Design review of the part built by this model. Coordinates are the model's own, in mm. Coordinates: 2 decimals unless noted, no trailing zeros. Order: outer loops, then holes, each group sorted by start corner. A loop starts at its lowest first (then second) coordinate and runs counter-clockwise, first axis right, second up. Notation, with made-up numbers: (24.25, 81) -> (82.25, 81) arc R19 ccw to (82.25, 114) -> close; hole circle Ø7 at (-13.5, 16.25). An arc over 180 degrees is marked (long way). Write item = value, one per line.
```python
from build123d import *

# Parameters (mm, degrees)
BOSS_EXTRUDE1_DEPTH = 6.35
SKETCH2_R           = 6.35
CUT_EXTRUDE1_DEPTH  = 6.35
CUT_EXTRUDE4_DEPTH  = 6.35


with BuildPart() as part:
    # Sketch1 → Boss-Extrude1 (new body)
    with BuildSketch(Plane.XY):
        Polygon((20.505148302, 25.897062134), (-23.613528139, 31.314154449), (25.914173021, 434.684910476), (95.764173021, 434.684910476), (95.764173021, 95.747062134), (29.081649881, 95.747062134), align=None)
    extrude(amount=BOSS_EXTRUDE1_DEPTH)

    # Sketch2 → Cut-Extrude1 (cut)
    with BuildSketch(Plane.XY.offset(6.35)):
        with Locations((72.594859494, 436.135448726)):
            Circle(SKETCH2_R)
    extrude(amount=-CUT_EXTRUDE1_DEPTH, mode=Mode.SUBTRACT)

    # Sketch4 → Cut-Extrude4 (cut)
    with BuildSketch(Plane.XY.offset(6.35)):
        with BuildLine():
            Line((74.295018445, 431.943320697), (82.016159891, 440.361424689))
            Line((82.016159891, 440.361424689), (105.989857785, 438.164600241))
            Line((105.989857785, 438.164600241), (95.764173021, 334.935994434))
            ThreePointArc((95.764173021, 334.935994434), (92.231289046, 356.088107858), (82.016159891, 374.943990437))
            ThreePointArc((82.016159891, 374.943990437), (70.461962448, 402.401475249), (74.295018445, 431.943320697))
        make_face()
    extrude(amount=-CUT_EXTRUDE4_DEPTH, mode=Mode.SUBTRACT)


solid = part.part
```
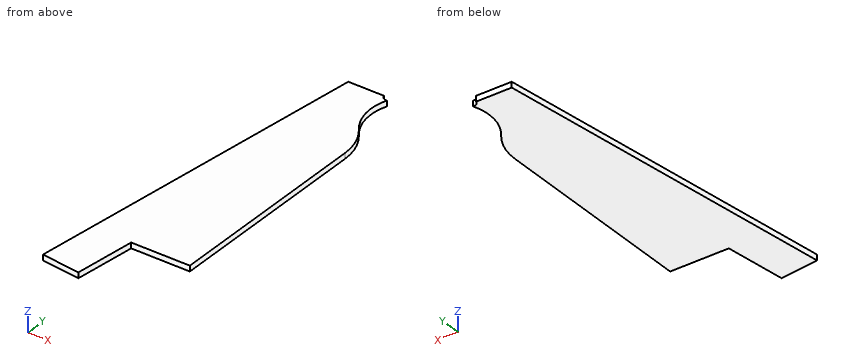
(1) Insertion check: pin 1 (2 mm diameter, centred on x = 56, z = 3, fed in from -Y). The pin has a flat end and moves straight along its axis. Give the tip position at first contact, or say it passes through.
Report:
pin_1 = 95.75
(2) For L1, parallel to Y at x = 43, z = 2; L2, parallel to Y at x = 82, z = 4.5; L3, parallel to X at y = 413.5, z = 0.5, list the stretches that pass through material, from the lowest coordinate up.
Report:
L1 = 95.75 to 434.68
L2 = 95.75 to 374.96
L3 = 23.31 to 70.05
(3) We need section B-B (x = 63). Write out the cut boundary in (y, z).
Report:
outline = (95.75, 0) -> (434.68, 0) -> (434.68, 6.35) -> (95.75, 6.35) -> close
(4) We need section C-C (y = 228). Write out the cut boundary in (x, z), and give its area (3 significant figures).
Report:
outline = (0.54, 0) -> (95.76, 0) -> (95.76, 6.35) -> (0.54, 6.35) -> close
area = 605 mm²
